Design review of the part built by this model. Coordinates are the model's own, in mm. Round coordinates to 2 decimals unless told otherwise and drop trailing zeros. Order: outer loops, then holes, each group sorted by start corner. A loop starts at its lowest first (then second) coordinate and runs counter-clockwise, first axis right, second up. Notation, with made-up numbers: M 45.25,56 L 54.25,56 A22 ccw 54.25,64 Z; hole C -36.5,-22.5 d2. An arc over 180 degrees is marked long. Use a Markdown table: item, result. Add a question column.
(1) To check wall thickness, follow probe 1 along X at (y, z) = (0.25, -29); probe 2 along Z at (x, y) = (-47, 2.8); probe 3 along X at (y, z) = (2.2, -58). State the ranges of each line that lie inside material, in increasing order. Write a range as from..to.
(2) Take a section at B-B (x = 18). Write out the cut boundary in (y, z), then the cut area to 3 significant figures.
(3) The part is to be moulded in two halves that separate along X. For faces 1 (the face through (-1, 1, 0)), 2 (the face through (66.36, 1.52, -47.91)), say which applies: released by +X, released by -X, zero draft, split by the parting line, or undercut.
(4) Take a section at C-C (y = 2.55). Count the separate pieces of the cut face and the enclosed holes in it, then the cut area to 3 significant figures.
(5) Take a section at A-A (x = -57.5). Write out the cut boundary in (y, z).
(6) For pin 1 (1.5 mm diameter, centred on x = 4, y = 2, fed in from +Z); pin 2 (1 mm diameter, centred on x = 37.5, z = -37.5, fed in from +Y); pin 3 (1.5 mm diameter, centred on y = 1, z = -9.5, fed in from +X); pin 4 (1.5 mm diameter, centred on y = 1, z = -39, fed in from +X), all flat-tipped, find the tip position at first contact; note any pin that passes through.
```python
from build123d import *

# Parameters (mm, degrees)
BOSS_EXTRUDE1_DEPTH = 3
CUT_EXTRUDE1_DEPTH  = 10
SKETCH3_W           = 3
SKETCH3_H           = 30
CUT_EXTRUDE2_DEPTH  = 10
SKETCH4_R           = 5.072960447
SKETCH4_R_2         = 3
SKETCH4_R_3         = 5.296326198
SKETCH4_R_4         = 6.795684495
CUT_EXTRUDE3_DEPTH  = 10


with BuildPart() as part:
    # Sketch1 → Boss-Extrude1 (new body)
    with BuildSketch(Plane(origin=(0, 0, 0), x_dir=(1, 0, 0), z_dir=(0, 1, 0))):
        Polygon((-72.98636562, 0), (72.98636562, 0), (74.075, 77), (-74.075, 77), align=None)
    extrude(amount=BOSS_EXTRUDE1_DEPTH)

    # Sketch2 → Cut-Extrude1 (cut)
    with BuildSketch(Plane(origin=(0, 3, 0), x_dir=(1, 0, 0), z_dir=(0, 1, 0))):
        with BuildLine():
            Line((-46.75, 63), (-53.876067096, 63))
            ThreePointArc((-53.876067096, 63), (-60.947134908, 60.071067812), (-63.876067096, 53))
            Line((-63.876067096, 53), (-63.876067096, 20))
            ThreePointArc((-63.876067096, 20), (-60.947134908, 12.928932188), (-53.876067096, 10))
            Line((-53.876067096, 10), (-46.75, 10))
            ThreePointArc((-46.75, 10), (-39.678932188, 12.928932188), (-36.75, 20))
            Line((-36.75, 20), (-36.75, 53))
            ThreePointArc((-36.75, 53), (-39.678932188, 60.071067812), (-46.75, 63))
        make_face()
        with BuildLine():
            Line((-13.25, 63), (0, 63))
            Line((0, 63), (0, 10))
            Line((0, 10), (-13.25, 10))
            ThreePointArc((-13.25, 10), (-20.321067812, 12.928932188), (-23.25, 20))
            Line((-23.25, 20), (-23.25, 53))
            ThreePointArc((-23.25, 53), (-20.321067812, 60.071067812), (-13.25, 63))
        make_face()
    cut_extrude1 = extrude(amount=-CUT_EXTRUDE1_DEPTH, mode=Mode.SUBTRACT)

    # Mirror1: Cut-Extrude1 across plane
    add(cut_extrude1.mirror(Plane(origin=(0, 0, 0), x_dir=(0, 0, 1), z_dir=(1, 0, 0))), mode=Mode.SUBTRACT)

    # Sketch3 → Cut-Extrude2 (cut)
    with BuildSketch(Plane(origin=(0, 3, 0), x_dir=(1, 0, 0), z_dir=(0, 1, 0))):
        with Locations((-28.5, 37)):
            Rectangle(SKETCH3_W, SKETCH3_H)
        with Locations((28.5, 37)):
            Rectangle(SKETCH3_W, SKETCH3_H)
    extrude(amount=-CUT_EXTRUDE2_DEPTH, mode=Mode.SUBTRACT)

    # Sketch4 → Cut-Extrude3 (cut)
    with BuildSketch(Plane(origin=(0, 3, 0), x_dir=(1, 0, 0), z_dir=(0, 1, 0))):
        with Locations((-65.508622451, 68.795423202)):
            Circle(SKETCH4_R)
        with Locations((-68.571363241, 57.565373639)):
            Circle(SKETCH4_R_2)
        with Locations((-68.571363241, 45.881584699)):
            Circle(SKETCH4_R_2)
        with Locations((-68.571363241, 33.403751851)):
            Circle(SKETCH4_R_2)
        with Locations((-68.571363241, 22.287137133)):
            Circle(SKETCH4_R_2)
        with Locations((-51.55613663, 5.385345366)):
            Circle(SKETCH4_R_2)
        with Locations((-41.460435508, 5.385345366)):
            Circle(SKETCH4_R_2)
        with Locations((-16.618204656, 5.385345366)):
            Circle(SKETCH4_R_2)
        with Locations((-5.84189447, 5.385345366)):
            Circle(SKETCH4_R_2)
        with Locations((-65.508622451, 7.880911935)):
            Circle(SKETCH4_R_3)
        with Locations((-29.209472348, 10.149608817)):
            Circle(SKETCH4_R_4)
        with Locations((29.209472348, 10.149608817)):
            Circle(SKETCH4_R_4)
        with Locations((65.508622451, 7.880911935)):
            Circle(SKETCH4_R_3)
        with Locations((5.84189447, 5.385345366)):
            Circle(SKETCH4_R_2)
        with Locations((16.618204656, 5.385345366)):
            Circle(SKETCH4_R_2)
        with Locations((41.460435508, 5.385345366)):
            Circle(SKETCH4_R_2)
        with Locations((51.55613663, 5.385345366)):
            Circle(SKETCH4_R_2)
        with Locations((68.571363241, 22.287137133)):
            Circle(SKETCH4_R_2)
        with Locations((68.571363241, 33.403751851)):
            Circle(SKETCH4_R_2)
        with Locations((68.571363241, 45.881584699)):
            Circle(SKETCH4_R_2)
        with Locations((68.571363241, 57.565373639)):
            Circle(SKETCH4_R_2)
        with Locations((65.508622451, 68.795423202)):
            Circle(SKETCH4_R)
    extrude(amount=-CUT_EXTRUDE3_DEPTH, mode=Mode.SUBTRACT)


solid = part.part
```
Verdict:
| question | item | result |
|---|---|---|
| 1 | probe 1 | x = -73.4..-63.88, -36.75..-30, -27..-23.25, 23.25..27, 30..36.75, 63.88..73.4 |
| 1 | probe 2 | z = -77..-63, -10..0 |
| 1 | probe 3 | x = -73.81..-71.54, -65.6..-62.54, -38.09..-21.91, 21.91..38.09, 62.54..65.6, 71.54..73.81 |
| 2 | outline | M 0,-77 L 3,-77 L 3,-61.8 L 0,-61.8 Z; M 0,-11.2 L 3,-11.2 L 3,-8.05 L 0,-8.05 Z; M 0,-2.72 L 3,-2.72 L 3,0 L 0,0 Z |
| 2 | area | 63.2 mm^2 |
| 3 | face 1 | zero draft |
| 3 | face 2 | undercut |
| 4 | separate pieces | 1 |
| 4 | enclosed holes | 27 |
| 4 | area | 4,980 mm^2 |
| 5 | outline | M 0,-77 L 3,-77 L 3,-62.32 L 0,-62.32 Z; M 0,-10.68 L 3,-10.68 L 3,0 L 0,0 Z |
| 6 | pin 1 | stops at z = 0 |
| 6 | pin 2 | passes through |
| 6 | pin 3 | stops at x = 73.13 |
| 6 | pin 4 | stops at x = 73.55 |
